Geometry: final body of the model. Coordinates: model frame, mm. Face numbers are marked on the shaded views. A direction names the side the tool comes from. Round coordinates to 2 decimals unless told otherwise and drop trailing zeros. Loops run counter-clockwise (first coordinate to the right, second up) from the corner with the lowest first, then second, coordinate; pieces in that order, holes last. Notation, with made-up numbers: M 3,-29.75 L 18,-29.75 A16 cw 18,-13.75 Z; hole C 80.25,-17 d3. An arc over 180 degrees is marked long. Answer as a JSON object with one key per item and string values.
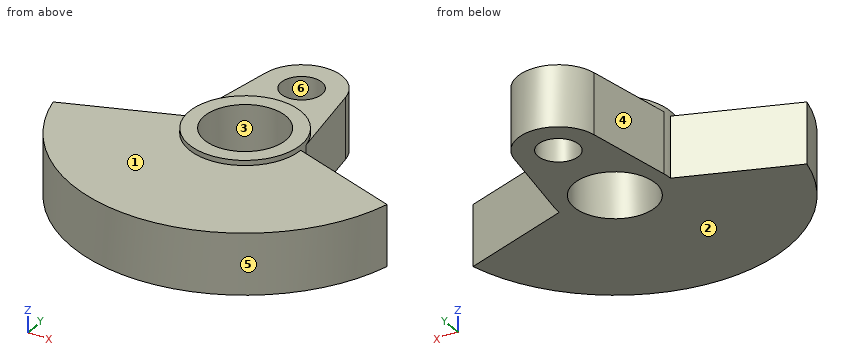
```python
from build123d import *

# Parameters (mm, degrees)
BOSS_EXTRUDE1_DEPTH   = 3
SKETCH1_R             = 2
BOSS_EXTRUDE1_2_DEPTH = 3
BOSS_EXTRUDE4_START   = 3.5
SKETCH1_6_R           = 5.5
SKETCH1_6_R_2         = 4
BOSS_EXTRUDE4_DEPTH   = 6.5
SCALE1_SCALE          = 1.5


with BuildPart() as part:
    # Sketch1 → Boss-Extrude1 (new, symmetric)
    with BuildSketch(Plane.XY):
        with BuildLine():
            Line((-5.5, 0), (-16.522711642, -4))
            ThreePointArc((-16.522711642, -4), (0, -17), (16.522711642, -4))
            Line((16.522711642, -4), (5.5, 0))
            ThreePointArc((5.5, 0), (0, -5.5), (-5.5, 0))
        make_face()
    extrude(amount=BOSS_EXTRUDE1_DEPTH, both=True)



with BuildPart() as body_2:
    # Sketch1 → Boss-Extrude1 2 (new, symmetric)
    with BuildSketch(Plane.XY):
        with BuildLine():
            Line((-3.944053189, 9.666666667), (-5.423073135, 0.916666667))
            ThreePointArc((-5.423073135, 0.916666667), (-0.058211757, 5.499691936), (5.402455316, 1.03125))
            Line((5.402455316, 1.03125), (3.944146954, 9.666111708))
            ThreePointArc((3.944146954, 9.666111708), (0.000281412, 12.99999999), (-3.944053189, 9.666666667))
        make_face()
        with Locations((0, 9)):
            Circle(SKETCH1_R, mode=Mode.SUBTRACT)
    extrude(amount=BOSS_EXTRUDE1_2_DEPTH, both=True)


with BuildPart() as part_1:
    add(part.part)

    add(body_2.part)  # Boss-Extrude4 merges body 2
    # Sketch1<6> → Boss-Extrude4 (add)
    with BuildSketch(Plane.XY.offset(BOSS_EXTRUDE4_START)):
        Circle(SKETCH1_6_R)
        with Locations(Location((0, 0, 0), (0, 0, 180))):
            Circle(SKETCH1_6_R_2, mode=Mode.SUBTRACT)
    extrude(amount=-BOSS_EXTRUDE4_DEPTH)


with BuildPart() as part_2:
    # Scale1: scaled about (-5.8229e-05, -5.841049103, 0.026355908)
    add(part_1.part.scale(SCALE1_SCALE).moved(Location((2.9115e-05, 2.920524551, -0.013177954))))


solid = part_2.part
```
1) Cut plane D-D on x = 5. Return the cut outline in (y, z).
Geometry results:
{"outline": "M -22.08,-4.51 L -0.4,-4.51 L -0.4,5.24 L -3.64,5.24 L -3.64,4.49 L -22.08,4.49 Z; M 6.24,-4.51 L 19.74,-4.51 L 19.74,4.49 L 9.48,4.49 L 9.48,5.24 L 6.24,5.24 Z"}
2) Cut plane B-B on x = -2. Return the cut outline in (y, z), and give its area (3 significant figures).
Geometry results:
{"outline": "M -22.5,-4.51 L -2.74,-4.51 L -2.74,5.24 L -5.08,5.24 L -5.08,4.49 L -22.5,4.49 Z; M 8.58,-4.51 L 14.18,-4.51 L 14.18,4.49 L 10.92,4.49 L 10.92,5.24 L 8.58,5.24 Z; M 18.66,-4.51 L 22.08,-4.51 L 22.08,4.49 L 18.66,4.49 Z", "area": "263 mm2"}
3) Cut plane C-C on z = -1.75. Return the cut outline in (x, y).
Geometry results:
{"outline": "M -24.78,-3.08 A25.5 ccw 24.78,-3.08 L 8.25,2.92 A8.25 ccw 8.1,4.47 L 5.92,17.42 A6 ccw -5.92,17.42 L -8.13,4.3 A8.25 ccw -8.25,2.92 Z; hole C 0,2.92 d12; hole C 0,16.42 d6"}
4) Line query: probe 1 along Y at (x, z) = (-2, 2.75); probe 2 along Z at (x, y) = (1, -13.5); probe 3 along Y at (x, z) = (-4, -1.5). Output: solid intervals per line, ascending.
Geometry results:
{"probe 1": "-22.5 to -2.74, 8.58 to 14.18, 18.66 to 22.08", "probe 2": "-4.51 to 4.49", "probe 3": "-22.26 to -1.55, 7.39 to 20.89"}
5) Set-up query: the marked faces 1 and 2. Return all of +Z, -Z, +X, -X, +Y, -Y with unobstructed straight access to the full face (end or side cutting, diameter ignored); none if empty.
Geometry results:
{"face 1": "+Z, -Y", "face 2": "-Z, +X, -X, +Y, -Y"}
6) Pull-direction query (Y, two-part tool) for the marked faces 3, 4, 5 and 6; classes: +Y half, -Y half, draft (parallel to the pull), parting line (faces both ways), or undercut.
Geometry results:
{"face 3": "undercut", "face 4": "+Y half", "face 5": "-Y half", "face 6": "undercut"}
7) First-contact query: pin 1 (3.5 mm diameter, centred on x = 0, y = 16.42, fed in from +Z); pin 2 (2 mm diameter, centred on x = 14, z = -0.5, fed in from +Y); pin 3 (5 mm diameter, centred on y = 15, z = 0.5, fed in from +X); pin 4 (2 mm diameter, centred on x = -4, z = 4, fed in from -Y). Flat tips, straight axial feed; report the tip coordinate or a pass-through.
Geometry results:
{"pin 1": "through", "pin 2": "y = 1.2", "pin 3": "x = 6.75", "pin 4": "y = -22.4"}
8) Cut plane A-A on y = 0. Return the cut outline in (x, z).
Geometry results:
{"outline": "M -16.3,-4.51 L -5.24,-4.51 L -5.24,5.24 L -7.72,5.24 L -7.72,4.49 L -16.3,4.49 Z; M 5.24,-4.51 L 16.3,-4.51 L 16.3,4.49 L 7.72,4.49 L 7.72,5.24 L 5.24,5.24 Z"}
